Input: dimensioned drawing with shaded views. Units: mm. Origin: part minimum x, y, z. Round coordinates to 2 decimals unless told otherwise and drop trailing zeros. Loops run counter-clockwise (first coordinate to the right, second up) from the corner with the lowest first, then second, coordinate; pieces in that order, holes last. Notation, with made-up numbers: M -27,27.25 L -9,27.25 A22 cw -9,50.25 Z; hole C 21,-6 d3. An arc over 180 degrees is marked long. Use one line per item in the form item = value. Start each with the question number.
Q1. First-contact query: P1, Ø2, axis at y = 9, z = 16.5, coming from the -X side; P2, Ø8, axis at x = 44.5, y = 13.5, coming from the +Z side; P3, Ø12, axis at y = 38.5, z = 16.5, coming from the -X side; P4, Ø5, axis at x = 37, z = 6.5, coming from the +Y side. Flat tips, straight axial feed; report the tip coordinate or a pass-through.
Q2. Section query A-A, the plane z = 1.75. Output: boundary loops of the cut face in (x, y).
Q3. Ray query, line 1 along Y through (x, z) = (25, 2.9); line 2 along Y through (x, z) = (25, 21.75); line 3 along Y through (x, z) = (31.5, 17.25). Return the intervals inside material, ascending.
Q4. Mould query, pull axis X, two halves, no side actions, for the marked faces 1, 2 and 3. Classes: pulls with the +X half, pulls with the -X half, needs draft (parallel to the pull), parting line crosses it, or undercut.
Q5. Section query C-C, the plane y = 33. Output: boundary loops of the cut face in (x, z), and give its area (3 significant figures).
Q6. Section query B-B, the plane x = 25. Output: boundary loops of the cut face in (y, z), and give its area (3 significant figures).
Q7. Section query D-D, the plane x = 41.5. Output: boundary loops of the cut face in (y, z), and give its area (3 significant figures).
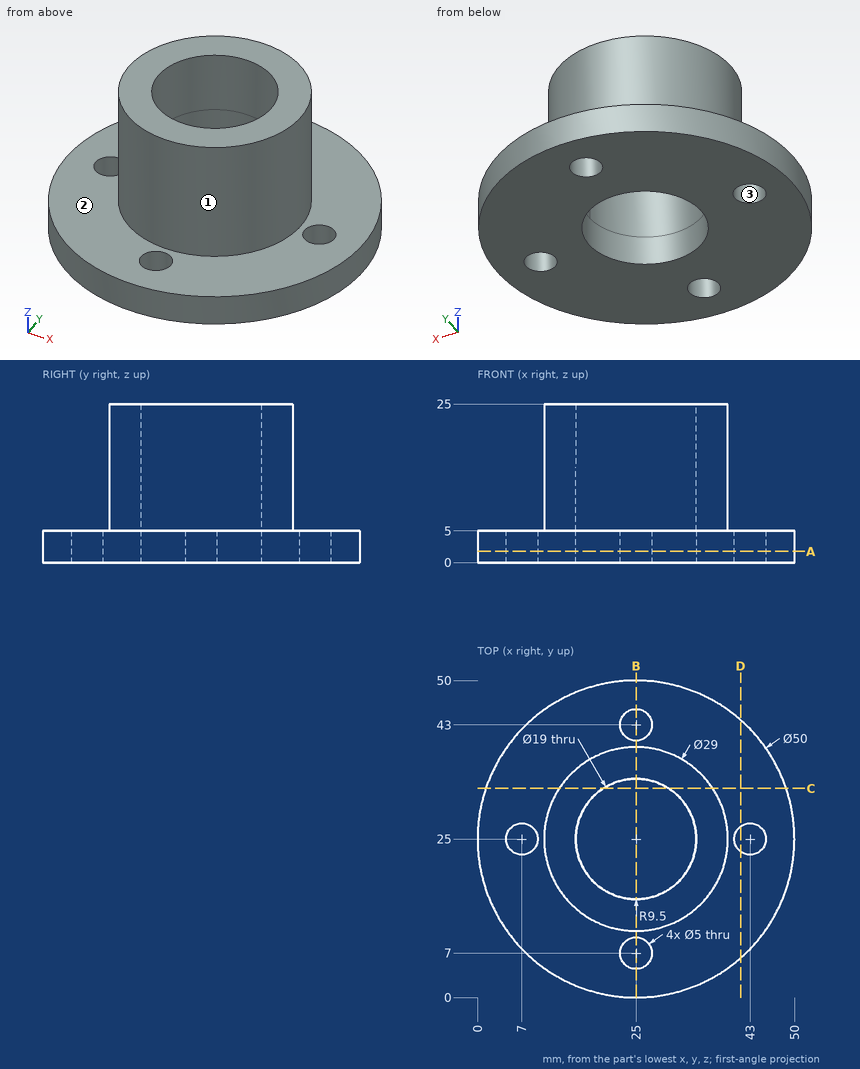
Results found:
q1.P1 = through
q1.P2 = 5
q1.P3 = 12.59
q1.P4 = 47.91
q2.outline = C 25,25 d50; hole C 7,25 d5; hole C 25,25 d19; hole C 25,7 d5; hole C 25,43 d5; hole C 43,25 d5
q3.line_1 = 0 to 4.5, 9.5 to 15.5, 34.5 to 40.5, 45.5 to 50
q3.line_2 = 10.5 to 15.5, 34.5 to 39.5
q3.line_3 = 12.04 to 18.07, 31.93 to 37.96
q4.face_1 = parting line crosses it
q4.face_2 = needs draft
q4.face_3 = undercut
q5.outline = M 1.31,0 L 19.88,0 L 19.88,25 L 12.91,25 L 12.91,5 L 1.31,5 Z; M 30.12,0 L 48.69,0 L 48.69,5 L 37.09,5 L 37.09,25 L 30.12,25 Z
q5.area = 464 mm²
q6.outline = M 0,0 L 4.5,0 L 4.5,5 L 0,5 Z; M 9.5,0 L 15.5,0 L 15.5,25 L 10.5,25 L 10.5,5 L 9.5,5 Z; M 34.5,0 L 40.5,0 L 40.5,5 L 39.5,5 L 39.5,25 L 34.5,25 Z; M 45.5,0 L 50,0 L 50,5 L 45.5,5 Z
q6.area = 305 mm²
q7.outline = M 6.22,0 L 23,0 L 23,5 L 6.22,5 Z; M 27,0 L 43.78,0 L 43.78,5 L 27,5 Z
q7.area = 168 mm²
